Can you work these out from the model? Positions are in its coordinate system, mm. Face numbers are marked on the shaded views. A direction names the side the tool comes from. Round coordinates to 2 decimals unless told otherwise and drop trailing zeros. Loops run counter-clockwise (first coordinate to the right, second up) from the corner with the lowest first, then second, coordinate; pieces in that order, holes last. Notation, with made-up numbers: M 15.5,24.25 L 55.5,24.25 A27 ccw 55.5,60.25 Z; hole C 29,0 d5. An arc over 180 degrees is marked long. Return JSON: item names as keys, results as strings.
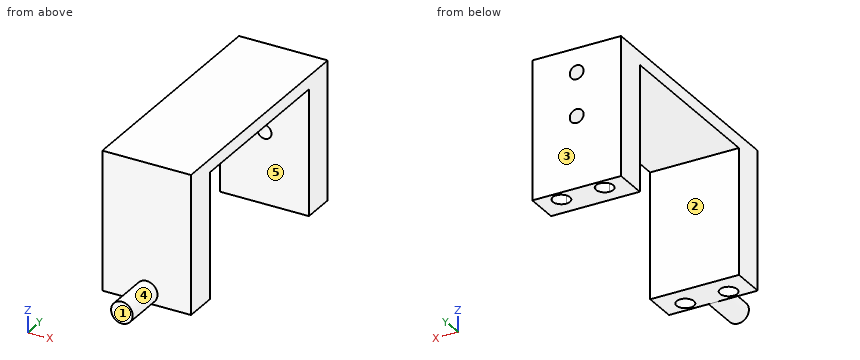
```python
from build123d import *

# Parameters (mm, degrees)
SKETCH_1_W          = 20.5
SKETCH_1_H          = 15.141704846
SKETCH_1_R          = 2
EXTRUDE_1_DEPTH     = 29
SKETCH_2_W          = 20.5
SKETCH_2_H          = 70.283409692
EXTRUDE_2_DEPTH     = 3
SKETCH_3_W          = 20.5
SKETCH_3_H          = 7.570852423
CUT_EXTRUDE_1_DEPTH = 49.621002864
SKETCH_5_R          = 2.5
EXTRUDE_3_DEPTH     = 10
CUT_EXTRUDE_2_REACH = 75.297
SKETCH_8_R          = 1.6


with BuildPart() as part:
    # 草图1 → 凸台-拉伸1 (new body)
    # profile 1 of 3: a face of its own
    with BuildSketch(Plane.XY):
        with BuildLine():
            Line((-10.25, 35.141704846), (-10.25, 20))
            Line((-10.25, 20), (-5, 20))
            Line((-5, 20), (-5, 23))
            ThreePointArc((-5, 23), (-6.414213562, 26.414213562), (-3, 25))
            Line((-3, 25), (3, 25))
            ThreePointArc((3, 25), (5, 27), (7, 25))
            ThreePointArc((7, 25), (6.414213562, 23.585786438), (5, 23))
            Line((5, 23), (5, 20))
            Line((5, 20), (10.25, 20))
            Line((10.25, 20), (10.25, 35.141704846))
            Line((10.25, 35.141704846), (-10.25, 35.141704846))
        make_face()
    # profile 2 of 3: a face of its own
    with BuildSketch(Plane.XY):
        with Locations((0, -27.570852423)):
            Rectangle(SKETCH_1_W, SKETCH_1_H)
        with Locations(Location((-5, -25, 0), (0, 0, 180))):
            Circle(SKETCH_1_R, mode=Mode.SUBTRACT)
        with Locations(Location((5, -25, 0), (0, 0, 180))):
            Circle(SKETCH_1_R, mode=Mode.SUBTRACT)
    # profile 3 of 3: a face of its own
    with BuildSketch(Plane.XY):
        with BuildLine():
            Line((-5, 23), (-5, 20))
            Line((-5, 20), (5, 20))
            Line((5, 20), (5, 23))
            ThreePointArc((5, 23), (3.585786438, 23.585786438), (3, 25))
            Line((3, 25), (-3, 25))
            ThreePointArc((-3, 25), (-3.585786438, 23.585786438), (-5, 23))
        make_face()
    extrude(amount=EXTRUDE_1_DEPTH)

    # 草图2 → 凸台-拉伸2 (add)
    with BuildSketch(Plane.XY.offset(29)):
        Rectangle(SKETCH_2_W, SKETCH_2_H)
    extrude(amount=EXTRUDE_2_DEPTH)

    # 草图3 → 切除-拉伸1 (cut, through all)
    with BuildSketch(Plane(origin=(0, 0, 0), x_dir=(-1, 0, 0), z_dir=(0, 0, -1))):
        with Locations((0, -31.356278635)):
            Rectangle(SKETCH_3_W, SKETCH_3_H)
        with Locations((0, 31.356278635)):
            Rectangle(SKETCH_3_W, SKETCH_3_H)
    extrude(amount=-CUT_EXTRUDE_1_DEPTH, mode=Mode.SUBTRACT)

    # 草图5 → 凸台-拉伸3 (add)
    with BuildSketch(Plane.XZ.offset(27.570852423)):
        with Locations(Location((0, 2.5, 0), (0, 0, 270))):
            Circle(SKETCH_5_R)
    extrude(amount=EXTRUDE_3_DEPTH)

    # 草图8 → 切除-拉伸2 (cut, up to next)
    with BuildSketch(Plane(origin=(0, 27.570852423, 0), x_dir=(1, 0, 0), z_dir=(0, 1, 0)), mode=Mode.PRIVATE) as cut_extrude_2_sk1:
        with Locations(Location((0, -16.5, 0), (0, 0, 270))):
            Circle(SKETCH_8_R)
    cut_extrude_2_tool1 = extrude(cut_extrude_2_sk1.sketch, amount=-CUT_EXTRUDE_2_REACH, mode=Mode.PRIVATE) & part.part
    # 草图8 → 切除-拉伸2 (cut, up to next)
    with BuildSketch(Plane(origin=(0, 27.570852423, 0), x_dir=(1, 0, 0), z_dir=(0, 1, 0)), mode=Mode.PRIVATE) as cut_extrude_2_sk2:
        with Locations(Location((0, -26.5, 0), (0, 0, 270))):
            Circle(SKETCH_8_R)
    cut_extrude_2_tool2 = extrude(cut_extrude_2_sk2.sketch, amount=-CUT_EXTRUDE_2_REACH, mode=Mode.PRIVATE) & part.part
    add(cut_extrude_2_tool1.solids().sort_by_distance((0, 27.570852, 16.5))[0], mode=Mode.SUBTRACT)
    add(cut_extrude_2_tool2.solids().sort_by_distance((0, 27.570852, 26.5))[0], mode=Mode.SUBTRACT)


solid = part.part
```
Q1. If I drill on line 1 along X through (y, z) = (-25, 20); line 2 along Y through (x, z) = (5, 6.5); line 3 along Y through (x, z) = (-3.5, 5), over which ranges is the centre line in solid material (lowest first)?
Results:
{"line 1": "x = -10.25 to -7, -3 to 3, 7 to 10.25", "line 2": "y = -27.57 to -27, -23 to -20, 20 to 23, 27 to 27.57", "line 3": "y = -27.57 to -26.32, -23.68 to -20, 20 to 23.68, 26.32 to 27.57"}
Q2. I'm going to push flat-ended pins straight in: pin 1 Ø12 at (x, y) = (-6, -29) entering from +Z; pin 2 Ø4 at (x, z) = (2, 22.5) entering from -Y; pin 3 Ø2.5 at (x, y) = (5, -25) entering from -Z. Where does each tip first touch, or does it pass through?
Results:
{"pin 1": "stops at z = 32", "pin 2": "stops at y = -27.57", "pin 3": "stops at z = 29"}
Q3. Suppose I cut it at A-A, the plane z = 2.5. Please give me the cut outline in (x, y), plus the area to 3 significant figures.
Results:
{"outline": "M -10.25,-27.57 L -2.5,-27.57 L -2.5,-37.57 L 2.5,-37.57 L 2.5,-27.57 L 10.25,-27.57 L 10.25,-20 L -10.25,-20 Z; M -10.25,20 L 10.25,20 L 10.25,27.57 L -10.25,27.57 Z; hole C -5,-25 d4; hole C -5,25 d4; hole C 5,-25 d4; hole C 5,25 d4", "area": "310 mm2"}
Q4. On a 3-axis mill with a long thin cutter (end or side, diameter ignored), from which of +Z, -Z, +X, -X, +Y, -Y can I reach the whole of each face in a straight line? I mean the marked faces 1 and 2. Say none if no direction works.
Results:
{"face 1": "+Z, -Z, +X, -X, -Y", "face 2": "-Z, +X, -X"}
Q5. Suppose I cut it at D-D, the plane z = 8. Please give me the cut outline in (x, y).
Results:
{"outline": "M -10.25,-27.57 L 10.25,-27.57 L 10.25,-20 L -10.25,-20 Z; M -10.25,20 L 10.25,20 L 10.25,27.57 L -10.25,27.57 Z; hole C -5,-25 d4; hole C -5,25 d4; hole C 5,-25 d4; hole C 5,25 d4"}
Q6. Suppose I cut it at C-C, the plane y = -25. Please give me the cut outline in (x, z), plus the area to 3 significant figures.
Results:
{"outline": "M -10.25,0 L -7,0 L -7,29 L -3,29 L -3,0 L 3,0 L 3,29 L 7,29 L 7,0 L 10.25,0 L 10.25,32 L -10.25,32 Z", "area": "424 mm2"}
Q7. Thinking about a two-plate mould opening in Y: for the marked faces 3, 4 and 5, which applies, pulls with the +Y half, pulls with the -Y half, needs draft (parallel to the pull), parting line crosses it, or undercut?
Results:
{"face 3": "pulls with the +Y half", "face 4": "needs draft", "face 5": "undercut"}
Q8. Suppose I cut it at B-B, the plane z = 16.5. Please give me the cut outline in (x, y).
Results:
{"outline": "M -10.25,-27.57 L 10.25,-27.57 L 10.25,-20 L -10.25,-20 Z; M -10.25,20 L -1.6,20 L -1.6,27.57 L -10.25,27.57 Z; M 1.6,20 L 10.25,20 L 10.25,27.57 L 1.6,27.57 Z; hole C -5,-25 d4; hole C -5,25 d4; hole C 5,-25 d4; hole C 5,25 d4"}
